The drawing under review shows one solid part. Ordinate dimensions are in mm from its lowest x, y, z. A direction names the side the tool comes from. Give positions to 0.01 mm unless a question says otherwise; leave off trailing zeros. Loops run counter-clockwise (first coordinate to the right, second up) from the corner with the lowest first, then second, coordinate; pieces in that order, holes last. Notation, with made-up numbers: (84.5, 51.25) - (109.5, 51.25) arc R27 cw to (109.5, 77.25) - close; hole circle Ø5 at (-11, -13.75). An arc over 180 degrees is marked (long way). Write each question's results on one line, items separated by ' | '.
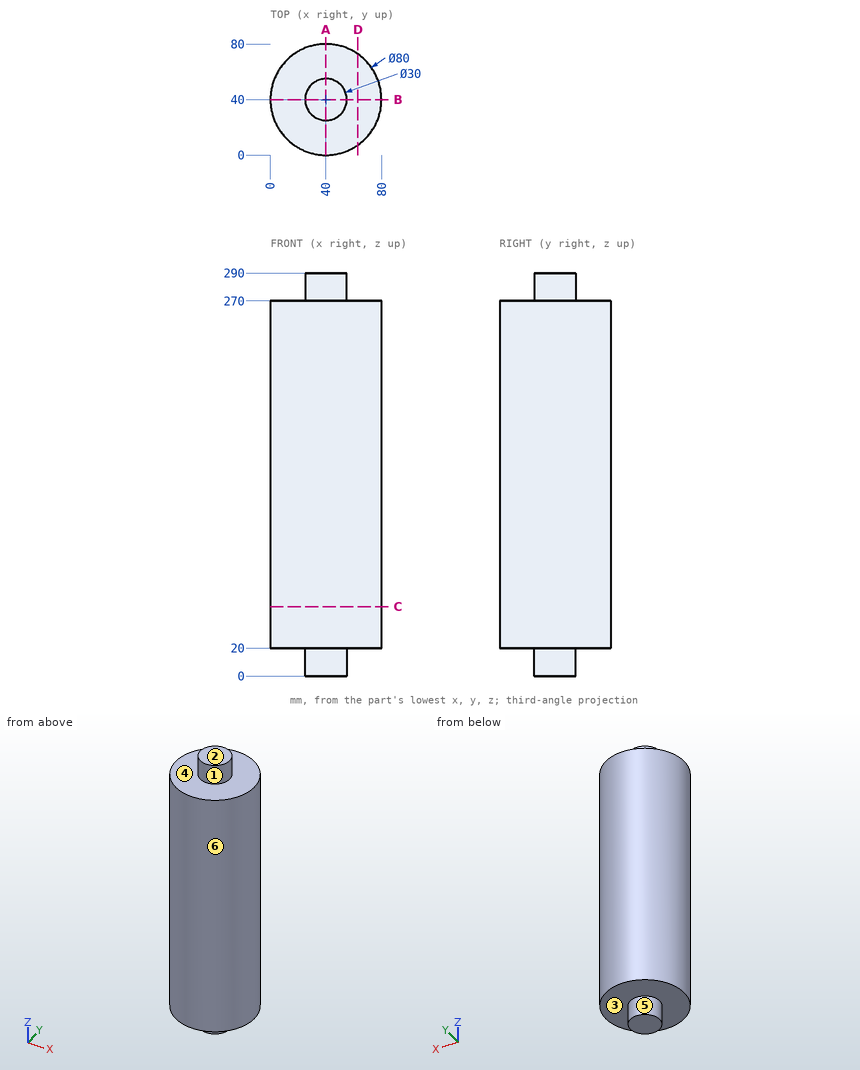
(1) Take a section at D-D on x = 63. Give the boundary of the cut face in (y, z).
Answers below:
outline: (7.27, 20) - (72.73, 20) - (72.73, 270) - (7.27, 270) - close
(2) Draft analysis for pull direction Z (two halves, no side actions). For the marked faces 1, 2 and 3, state which applies: pulls with the +Z half, pulls with the -Z half, needs draft (parallel to the pull), parting line crosses it, or undercut.
Answers below:
face 1: needs draft | face 2: pulls with the +Z half | face 3: pulls with the -Z half
(3) Take a section at A-A on x = 40. Give the boundary of the cut face in (y, z), plus the area to 3 significant figures.
Answers below:
outline: (0, 20) - (25, 20) - (25, 0) - (55, 0) - (55, 20) - (80, 20) - (80, 270) - (55, 270) - (55, 290) - (25, 290) - (25, 270) - (0, 270) - close | area: 21,200 mm2
(4) Insertion check: P1, Ø8, axis at x = 56.5, y = 62.5, coming from the -Z side; P2, Ø2, axis at x = 61.5, z = 48.5, coming from the -Y side; P3, Ø12, axis at x = 58.5, y = 70, coming from the +Z side; P4, Ø1.5, axis at x = 55, y = 37, coming from the -Z side. Each pin has a flat end and moves straight along its axis. Give the tip position at first contact, or say it passes through.
Answers below:
P1: z = 20 | P2: y = 5.65 | P3: z = 270 | P4: z = 0
(5) Tool access review of the marked faces 4, 5 and 6: name each direction out of +Z, -Z, +X, -X, +Y, -Y from which nothing blocks a thin tool from reaching the whole face with its end or side.
Answers below:
face 4: +Z | face 5: -Z | face 6: +Z, -Z
(6) Take a section at C-C on z = 50. Give the boundary of the cut face in (x, y).
Answers below:
outline: circle Ø80 at (40, 40)
(7) Wall thickness on line 1 along Z through (x, y) = (60, 34.5); line 2 along Y through (x, z) = (41, 60); line 3 along X through (y, z) = (23.5, 230): over which ranges is each line inside the solid? List them lowest first. Write a range as from..to.
Answers below:
line 1: 20..270 | line 2: 0.01..79.99 | line 3: 3.56..76.44
